Could you check a few things on this model? Use its own coordinates, in mm. A direction names the side the tool comes from. Round coordinates to 2 decimals unless told otherwise and drop trailing zeros. Loops run counter-clockwise (first coordinate to the right, second up) from the corner with the lowest first, then second, coordinate; pieces in that order, holes last. Notation, with made-up numbers: (49, 87) -> (105, 87) arc R19 cw to (105, 107) -> close; hole circle Ø5 at (84.25, 28.25). An arc over 180 degrees is marked (long way). One line per item, written item: value.
from build123d import *

# Parameters (mm, degrees)
SKETCH1_W           = 450
SKETCH1_H           = 500
BOSS_EXTRUDE1_DEPTH = 10
SKETCH2_W           = 450
SKETCH2_H           = 500
SKETCH2_W_2         = 430
SKETCH2_H_2         = 480
BOSS_EXTRUDE2_DEPTH = 140
SKETCH3_R           = 115
CUT_EXTRUDE1_DEPTH  = 10
SKETCH5_W           = 200
SKETCH5_H           = 100
CUT_EXTRUDE3_DEPTH  = 369.272996566
SKETCH6_R           = 5
CUT_EXTRUDE4_DEPTH  = 10
CUT_EXTRUDE5_START  = -10
SKETCH7_R           = 5
CUT_EXTRUDE5_DEPTH  = 10
SKETCH8_W           = 206
SKETCH8_H           = 56
SKETCH8_W_2         = 200
SKETCH8_H_2         = 50
BOSS_EXTRUDE3_DEPTH = 100


with BuildPart() as part:
    # Sketch1 → Boss-Extrude1 (new body)
    with BuildSketch(Plane(origin=(0, 0, 0), x_dir=(1, 0, 0), z_dir=(0, 1, 0))):
        Rectangle(SKETCH1_W, SKETCH1_H)
    extrude(amount=BOSS_EXTRUDE1_DEPTH)

    # Sketch2 → Boss-Extrude2 (add)
    with BuildSketch(Plane(origin=(0, 10, 0), x_dir=(1, 0, 0), z_dir=(0, 1, 0))):
        Rectangle(SKETCH2_W, SKETCH2_H)
        Rectangle(SKETCH2_W_2, SKETCH2_H_2, mode=Mode.SUBTRACT)
    extrude(amount=BOSS_EXTRUDE2_DEPTH)

    # Sketch3 → Cut-Extrude1 (cut)
    with BuildSketch(Plane(origin=(0, 10, 0), x_dir=(1, 0, 0), z_dir=(0, 1, 0))):
        with Locations(Location((0, 0, 0), (0, 0, 270))):
            Circle(SKETCH3_R)
    extrude(amount=-CUT_EXTRUDE1_DEPTH, mode=Mode.SUBTRACT)

    # Sketch5 → Cut-Extrude3 (cut, through all)
    with BuildSketch(Plane(origin=(0, 150, 0), x_dir=(1, 0, 0), z_dir=(0, 1, 0))):
        with Locations((0, -250)):
            Rectangle(SKETCH5_W, SKETCH5_H)
    extrude(amount=-CUT_EXTRUDE3_DEPTH, mode=Mode.SUBTRACT)

    # Sketch6 → Cut-Extrude4 (cut)
    with BuildSketch(Plane(origin=(225, 0, 0), x_dir=(0, 0, -1), z_dir=(1, 0, 0))):
        with Locations((-99.9, 34.7)):
            Circle(SKETCH6_R)
        with Locations((0.1, 33.13)):
            Circle(SKETCH6_R)
        with Locations((100.1, 33.13)):
            Circle(SKETCH6_R)
    extrude(amount=-CUT_EXTRUDE4_DEPTH, mode=Mode.SUBTRACT)

    # Sketch7 → Cut-Extrude5 (cut)
    with BuildSketch(Plane.ZY.offset(225).offset(CUT_EXTRUDE5_START)):
        with Locations(Location((-100.1, 33.13, 0), (0, 0, 180))):
            Circle(SKETCH7_R)
        with Locations(Location((-0.1, 33.13, 0), (0, 0, 180))):
            Circle(SKETCH7_R)
        with Locations(Location((99.9, 34.7, 0), (0, 0, 180))):
            Circle(SKETCH7_R)
    extrude(amount=CUT_EXTRUDE5_DEPTH, mode=Mode.SUBTRACT)

    # Sketch8 → Boss-Extrude3 (add)
    with BuildSketch(Plane(origin=(0, 10, 0), x_dir=(1, 0, 0), z_dir=(0, 1, 0))):
        with Locations((0, 195)):
            Rectangle(SKETCH8_W, SKETCH8_H)
        with Locations((0, 195)):
            Rectangle(SKETCH8_W_2, SKETCH8_H_2, mode=Mode.SUBTRACT)
    extrude(amount=BOSS_EXTRUDE3_DEPTH)


solid = part.part
(1) If I drill on L1, parallel to X at y = 20.5, z = -183; L2, parallel to Z at x = 80.5, y = 85.5; L3, parallel to Z at x = 101.5, y = 103.5, over which ranges is the centre line in solid material (lowest first)?
Recorded:
L1: -225 to -215, -103 to -100, 100 to 103, 215 to 225
L2: -250 to -240, -223 to -220, -170 to -167
L3: -250 to -240, -223 to -167, 240 to 250
(2) If we section it at A-A, the plane y = 67.5: Please give me the cut outline in (x, z).
Recorded:
outline: (-225, -250) -> (225, -250) -> (225, 250) -> (100, 250) -> (100, 240) -> (215, 240) -> (215, -240) -> (-215, -240) -> (-215, 240) -> (-100, 240) -> (-100, 250) -> (-225, 250) -> close; (-103, -223) -> (103, -223) -> (103, -167) -> (-103, -167) -> close; hole (-100, -220) -> (100, -220) -> (100, -170) -> (-100, -170) -> close
(3) For faces 1 (the face through (-100, 59, 242)), 2 (the face through (-158, 79, 240)), 3 (the face through (-112.265, 5.07, -24.93)), which set-ups out of +Z, -Z, +X, -X, +Y, -Y let a thin tool reach every point of the face, with its end or its side?
Recorded:
face 1: +Z, +Y, -Y
face 2: +Y
face 3: +Y, -Y
(4) If we section it at C-C, the plane z = -157: Please give me the cut outline in (x, y).
Recorded:
outline: (-225, 0) -> (225, 0) -> (225, 150) -> (215, 150) -> (215, 10) -> (-215, 10) -> (-215, 150) -> (-225, 150) -> close
(5) Thinking about a two-plate mould opening in X: for faces 4 (the face through (-215, 79, 3)), 5 (the face through (-163, 74, 250)), which applies, released by +X, released by -X, zero draft, split by the parting line, or undercut?
Recorded:
face 4: undercut
face 5: zero draft
(6) I'm going to push flat-ended pins straight in: pin 1 Ø16 at (y, z) = (33.13, -0.1) entering from -X; pin 2 Ø3 at (x, y) = (-9, 6) entering from +Z; pin 3 Ø3 at (x, z) = (-94.5, -189.5) entering from +Y. Where does each tip first touch, or does it pass through?
Recorded:
pin 1: x = -225
pin 2: z = 200
pin 3: y = 10
(7) If we section it at D-D, the plane y = 117.5: Please give me the cut outline in (x, z), then the cut area to 3 significant figures.
Recorded:
outline: (-225, -250) -> (225, -250) -> (225, 250) -> (100, 250) -> (100, 240) -> (215, 240) -> (215, -240) -> (-215, -240) -> (-215, 240) -> (-100, 240) -> (-100, 250) -> (-225, 250) -> close
area: 16,600 mm²
(8) If we section it at B-B, the plane x = -53: Please give me the cut outline in (y, z).
Recorded:
outline: (0, -250) -> (150, -250) -> (150, -240) -> (10, -240) -> (10, -223) -> (110, -223) -> (110, -220) -> (10, -220) -> (10, -170) -> (110, -170) -> (110, -167) -> (10, -167) -> (10, -102.06) -> (0, -102.06) -> close; (0, 102.06) -> (10, 102.06) -> (10, 200) -> (0, 200) -> close
